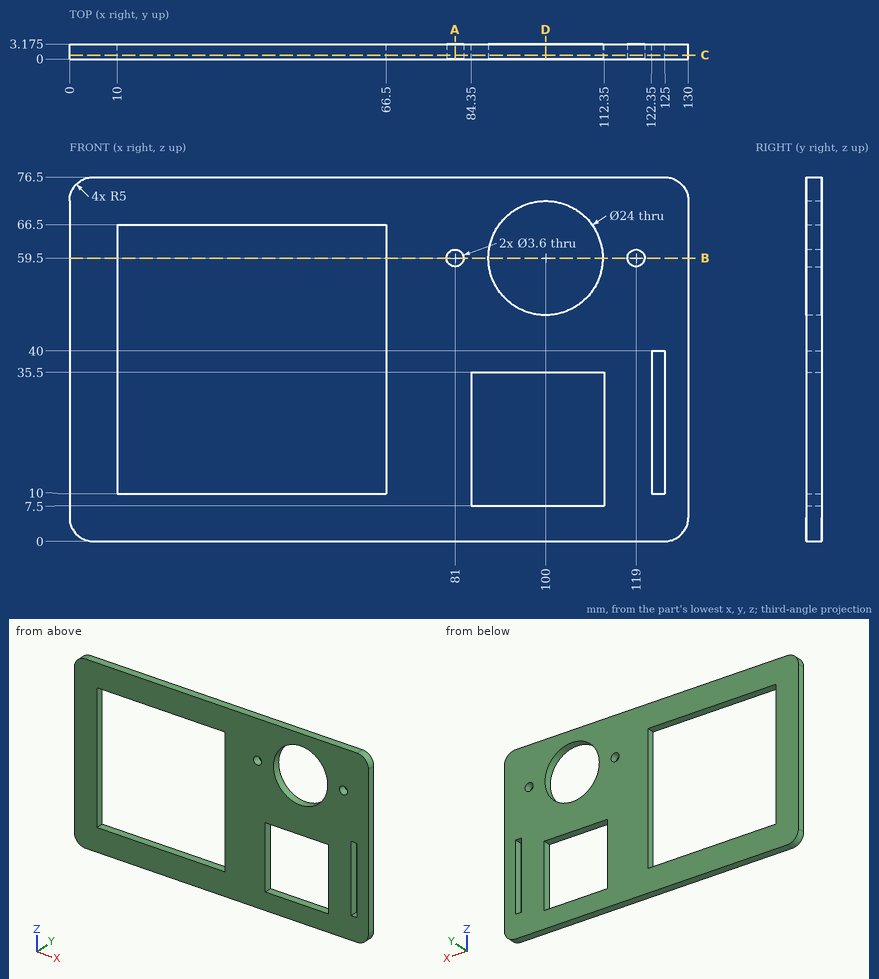
The figure shows three views and two pictorial views of one solid part (mm, origin at its lowest corner). Answer the questions. Round coordinates to 2 decimals unless told otherwise and drop trailing zeros. Write each loop counter-clockwise with the first axis right and the second up, starting at its lowest first coordinate (ties: lowest second). Pieces come first, ordered by that corner, then holes. Notation, with made-up numbers: (-5, 89.25) -> (18, 89.25) arc R31 ccw to (18, 127.25) -> close; hole circle Ø7 at (39.25, 3.5). An arc over 180 degrees is marked (long way). Answer as a JSON object with one key per item and string values. Group by question number.
Q1. Section A-A (x = 81) is taken. Write down the section's boundary in (y, z) (3 decimals).
Q2. Section C-C (y = 0.85) is taken. Write down the section's boundary in (x, z).
Q3. Section B-B (z = 59.5) is taken. Write down the section's boundary in (x, y) (3 decimals), plus the area to 3 significant figures.
Q4. Section D-D (x = 100) is taken. Write down the section's boundary in (y, z) (3 decimals).
Q5. Straight lines are drawn through the part: line 1 along X through (y, z) = (0.6, 19.5); line 2 along X through (y, z) = (1.1, 59.5); line 3 along Z through (x, y) = (14, 2.4). For each, find the intervals that lie inside material, in ascending order.
Check values:
{
 "1": {"outline": "(0, 0) -> (3.175, 0) -> (3.175, 57.7) -> (0, 57.7) -> close; (0, 61.3) -> (3.175, 61.3) -> (3.175, 76.5) -> (0, 76.5) -> close"},
 "2": {"outline": "(0, 5) arc R5 ccw to (5, 0) -> (125, 0) arc R5 ccw to (130, 5) -> (130, 71.5) arc R5 ccw to (125, 76.5) -> (5, 76.5) arc R5 ccw to (0, 71.5) -> close; hole (10, 10) -> (66.5, 10) -> (66.5, 66.5) -> (10, 66.5) -> close; hole circle Ø3.6 at (81, 59.5); hole (84.35, 7.5) -> (112.35, 7.5) -> (112.35, 35.5) -> (84.35, 35.5) -> close; hole circle Ø24 at (100, 59.5); hole circle Ø3.6 at (119, 59.5); hole (122.35, 10) -> (125, 10) -> (125, 40) -> (122.35, 40) -> close"},
 "3": {"outline": "(0, 0) -> (10, 0) -> (10, 3.175) -> (0, 3.175) -> close; (66.5, 0) -> (79.2, 0) -> (79.2, 3.175) -> (66.5, 3.175) -> close; (82.8, 0) -> (88, 0) -> (88, 3.175) -> (82.8, 3.175) -> close; (112, 0) -> (117.2, 0) -> (117.2, 3.175) -> (112, 3.175) -> close; (120.8, 0) -> (130, 0) -> (130, 3.175) -> (120.8, 3.175) -> close", "area": "134 mm^2"},
 "4": {"outline": "(0, 0) -> (3.175, 0) -> (3.175, 7.5) -> (0, 7.5) -> close; (0, 35.5) -> (3.175, 35.5) -> (3.175, 47.5) -> (0, 47.5) -> close; (0, 71.5) -> (3.175, 71.5) -> (3.175, 76.5) -> (0, 76.5) -> close"},
 "5": {"line 1": "0 to 10, 66.5 to 84.35, 112.35 to 122.35, 125 to 130", "line 2": "0 to 10, 66.5 to 79.2, 82.8 to 88, 112 to 117.2, 120.8 to 130", "line 3": "0 to 10, 66.5 to 76.5"}
}
